Design review of the part built by this model. Coordinates are the model's own, in mm. Give positions to 0.01 mm unless a question says otherwise; leave off trailing zeros. Write each loop counter-clockwise with the first axis right and the second up, starting at its lowest first coordinate (ties: lowest second). Pieces come first, ordered by that corner, then holes. Notation, with made-up numbers: (31, 79) -> (69, 79) arc R22 cw to (69, 92) -> close; hole circle Ø3 at (3.5, 43.5). An arc over 180 degrees is marked (long way). Answer as a JSON object with one key per item and string values.
```python
from build123d import *

# Parameters (mm, degrees)
SALIENTE_EXTRUIR1_DEPTH = 0.5
CORTAR_EXTRUIR6_REACH   = 31.207
CROQUIS6_R              = 2.5


with BuildPart() as part:
    # Croquis1 → Saliente-Extruir1 (new body)
    with BuildSketch(Plane.XY):
        with BuildLine():
            Line((0, 0), (0, -1.5))
            Line((0, -1.5), (-1.1, -1.5))
            Line((-1.1, -1.5), (-1.1, -2.8))
            Line((-1.1, -2.8), (0, -2.8))
            Line((0, -2.8), (0, -4.9))
            Line((0, -4.9), (-1.6, -7.033333333))
            Line((-1.6, -7.033333333), (-1.6, -19.280056819))
            add(Edge.make_bspline(
                [(-4.695633314, -25.550391636), (-1.6, -22.281455624), (-1.6, -19.280056819)],
                knots=[4.71238898, 4.71238898, 4.71238898, 5.777895429, 5.777895429, 5.777895429], degree=2, weights=[1, 0.861411956, 1]))
            ThreePointArc((-4.695633314, -25.550391636), (-11.549653085, -23.432645639), (-5.7, -19.280056819))
            Line((-5.7, -19.280056819), (-5.7, -6.2))
            Line((-5.7, -6.2), (-3.3, -3))
            Line((-3.3, -3), (-3.3, 0))
            Line((-3.3, 0), (0, 0))
        make_face()
    extrude(amount=SALIENTE_EXTRUIR1_DEPTH)

    # Croquis6 → Cortar-Extruir6 (cut, up to next)
    with BuildSketch(Plane.XY.offset(0.5), mode=Mode.PRIVATE) as cortar_extruir6_sk1:
        with Locations((-7.6, -22.8)):
            Circle(CROQUIS6_R)
    cortar_extruir6_tool1 = extrude(cortar_extruir6_sk1.sketch, amount=-CORTAR_EXTRUIR6_REACH, mode=Mode.PRIVATE) & part.part
    add(cortar_extruir6_tool1.solids().sort_by_distance((-7.6, -22.8, 0.5))[0], mode=Mode.SUBTRACT)


solid = part.part
```
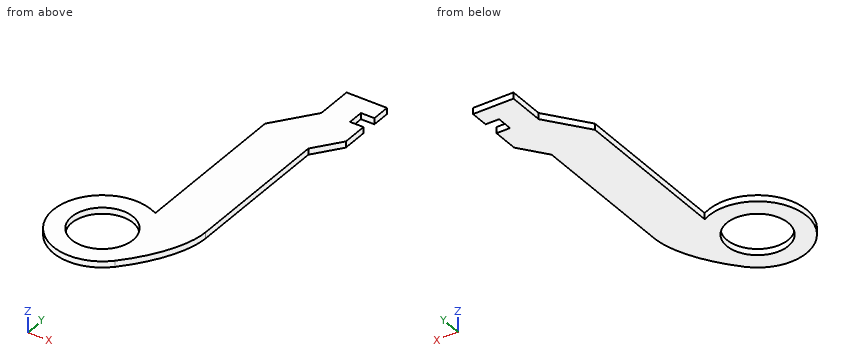
(1) For line 1 along Y through (x, z) = (-7.6, 0.35); line 2 along Y through (x, z) = (-9.25, 0.3); line 3 along X through (y, z) = (-21.75, 0.2), list the stretches that pass through material, from the lowest coordinate up.
Here are the results:
{"line 1": "y = -26.8 to -25.3, -20.3 to -18.8", "line 2": "y = -26.44 to -24.68, -20.92 to -19.16", "line 3": "x = -11.46 to -9.87, -5.33 to -2.16"}
(2) We need section A-A, the plane x = -7.6. State the section outline as (y, z) points, then the cut area to 3 significant figures.
Here are the results:
{"outline": "(-26.8, 0) -> (-25.3, 0) -> (-25.3, 0.5) -> (-26.8, 0.5) -> close; (-20.3, 0) -> (-18.8, 0) -> (-18.8, 0.5) -> (-20.3, 0.5) -> close", "area": "1.50 mm²"}
(3) Clearance check with a flat-ended pin moving along its axis: pin 1 (6 mm diameter, centred on x = -7.6, y = -22.8, fed in from -Z). State where the tip first meets the part, or that it passes through.
Here are the results:
{"pin 1": "stops at z = 0"}
(4) We need section B-B, the plane y = -16.25. State the section outline as (x, z) points.
Here are the results:
{"outline": "(-5.7, 0) -> (-1.6, 0) -> (-1.6, 0.5) -> (-5.7, 0.5) -> close"}
(5) We need section C-C, the plane y = -5.5. State the section outline as (x, z) points (3 decimals).
Here are the results:
{"outline": "(-5.175, 0) -> (-0.45, 0) -> (-0.45, 0.5) -> (-5.175, 0.5) -> close"}
